```python
from build123d import *

# Parameters (mm, degrees)
BOSS_EXTRUDE1_DEPTH = 3.175
FILLET1_R           = 3.175
FILLET2_R           = 1.5875
SKETCH3_W           = 3.175
SKETCH3_H           = 12.7
SKETCH3_W_2         = 12.7
SKETCH3_H_2         = 3.175
SKETCH3_W_3         = 6.35
BOSS_EXTRUDE2_DEPTH = 3.175
CUT_EXTRUDE1_DEPTH  = 282.187550651
FILLET3_R           = 0.3175


with BuildPart() as part:
    # Sketch1 → Boss-Extrude1 (new body)
    with BuildSketch(Plane.XY):
        Polygon((-276.225, 0), (276.225, 0), (276.225, 31.496), (263.525, 31.496), (251.079, 19.05), (-251.079, 19.05), (-263.525, 31.496), (-276.225, 31.496), align=None)
    extrude(amount=BOSS_EXTRUDE1_DEPTH)

    # Fillet1
    fillet1_edges = [part.edges().sort_by_distance(p)[0] for p in [
        (-263.525, 31.496, 1.5875),
        (-251.079, 19.05, 1.5875),
        (251.079, 19.05, 1.5875),
        (263.525, 31.496, 1.5875),
    ]]
    fillet(fillet1_edges, radius=FILLET1_R)

    # Fillet2
    fillet2_edges = [part.edges().sort_by_distance(p)[0] for p in [
        (-276.225, 31.496, 1.5875),
        (276.225, 31.496, 1.5875),
        (276.225, 0, 1.5875),
        (-276.225, 0, 1.5875),
    ]]
    fillet(fillet2_edges, radius=FILLET2_R)

    # Sketch3 → Boss-Extrude2 (add)
    with BuildSketch(Plane.XY.offset(3.175)):
        with Locations((277.8125, 15.748)):
            Rectangle(SKETCH3_W, SKETCH3_H)
        with Locations((138.1125, -1.5875)):
            Rectangle(SKETCH3_W_2, SKETCH3_H_2)
        with Locations((3.175, -1.5875)):
            Rectangle(SKETCH3_W_3, SKETCH3_H_2)
    boss_extrude2 = extrude(amount=-BOSS_EXTRUDE2_DEPTH)

    # Mirror1: Boss-Extrude2 across plane
    add(boss_extrude2.mirror(Plane(origin=(0, 0, 0), x_dir=(0, 0, 1), z_dir=(1, 0, 0))))

    # Sketch4 → Cut-Extrude1 (cut, through all)
    with BuildSketch(Plane.XY.offset(3.175)):
        with BuildLine():
            Line((-276.225, 22.733), (-275.59, 22.733))
            ThreePointArc((-275.59, 22.733), (-275.2725, 22.4155), (-275.59, 22.098))
            Line((-275.59, 22.098), (-276.225, 22.098))
            ThreePointArc((-276.225, 22.098), (-276.5425, 22.4155), (-276.225, 22.733))
        make_face()
        with BuildLine():
            Line((-276.225, 9.398), (-275.59, 9.398))
            ThreePointArc((-275.59, 9.398), (-275.2725, 9.0805), (-275.59, 8.763))
            Line((-275.59, 8.763), (-276.225, 8.763))
            ThreePointArc((-276.225, 8.763), (-276.5425, 9.0805), (-276.225, 9.398))
        make_face()
        with BuildLine():
            Line((-145.0975, 0), (-145.0975, 0.635))
            ThreePointArc((-145.0975, 0.635), (-144.78, 0.9525), (-144.4625, 0.635))
            Line((-144.4625, 0.635), (-144.4625, 0))
            ThreePointArc((-144.4625, 0), (-144.78, -0.3175), (-145.0975, 0))
        make_face()
        with BuildLine():
            Line((-131.1275, 0.635), (-131.1275, 0))
            ThreePointArc((-131.1275, 0), (-131.445, -0.3175), (-131.7625, 0))
            Line((-131.7625, 0), (-131.7625, 0.635))
            ThreePointArc((-131.7625, 0.635), (-131.445, 0.9525), (-131.1275, 0.635))
        make_face()
        with BuildLine():
            Line((-6.985, 0), (-6.985, 0.635))
            ThreePointArc((-6.985, 0.635), (-6.6675, 0.9525), (-6.35, 0.635))
            Line((-6.35, 0.635), (-6.35, 0))
            ThreePointArc((-6.35, 0), (-6.6675, -0.3175), (-6.985, 0))
        make_face()
    cut_extrude1 = extrude(amount=-CUT_EXTRUDE1_DEPTH, mode=Mode.SUBTRACT)

    # Mirror2: Cut-Extrude1 across plane
    add(cut_extrude1.mirror(Plane(origin=(0, 0, 0), x_dir=(0, 0, 1), z_dir=(1, 0, 0))), mode=Mode.SUBTRACT)

    # Fillet3
    fillet3_edges = [part.edges().sort_by_distance(p)[0] for p in [
        (-279.4, 22.098, 1.5875),
        (-279.4, 9.398, 1.5875),
        (-144.4625, -3.175, 1.5875),
        (-131.7625, -3.175, 1.5875),
        (-6.35, -3.175, 1.5875),
        (-276.225, 22.733, 1.5875),
        (-276.225, 8.763, 1.5875),
        (-145.0975, 0, 1.5875),
        (-131.1275, 0, 1.5875),
        (-6.985, 0, 1.5875),
        (276.225, 22.733, 1.5875),
        (276.225, 8.763, 1.5875),
        (145.0975, 0, 1.5875),
        (131.1275, 0, 1.5875),
        (6.985, 0, 1.5875),
        (279.4, 22.098, 1.5875),
        (279.4, 9.398, 1.5875),
        (131.7625, -3.175, 1.5875),
        (144.4625, -3.175, 1.5875),
        (6.35, -3.175, 1.5875),
    ]]
    fillet(fillet3_edges, radius=FILLET3_R)


solid = part.part
```
Here's how the part is built. I have some questions about the finished solid (model axes, mm). A direction names the side the tool comes from. Coordinates: 2 decimals unless noted, no trailing zeros. Order: outer loops, then holes, each group sorted by start corner. A loop starts at its lowest first (then second) coordinate and runs counter-clockwise, first axis right, second up.
1) Imagine slicing it at A-A on x = -222.5. List the corners of the cut face in (y, z) for me (3 decimals), and give its area (3 significant figures).
2) I need wall thicknesses on line 1 (Y direction, x = -46, z = 1.05); line 2 (Y direction, x = 137.5, z = 1.2) (3 decimals); line 3 (X direction, y = 24, z = 2.65) (3 decimals). Which ranges of each line are inside material? Lowest first, please.
3) Will these pins go through, and if not, where does the flat tip stop? pin 1 (1.6 mm diameter, centred on x = -94.5, z = 2, fed in from -Y); pin 2 (1 mm diameter, centred on x = -208.5, z = 1, fed in from +Y); pin 3 (1.6 mm diameter, centred on x = -278, z = 2, fed in from -Y).
4) We'd pull the mould along X, two halves only. Please class faces 1 (the face through (-257.23, 25.2, 1.57)), 2 (the face through (4, 11, 0)): +X half, -X half, draft (parallel to the pull), parting line (faces both ways), or undercut.
5) Which directions (+Z, -Z, +X, -X, +Y, -Y) give clear straight access to the entire face, cutting with the end or side of a thin tool? Please do faces 3 (the face through (4, 11, 3.175)), 4 (the face through (257.38, 25.35, 1.57)).
Response values:
1. outline: (0, 0) - (19.05, 0) - (19.05, 3.175) - (0, 3.175) - close
1. area: 60.5 mm2
2. line 1: y = 0 to 19.05
2. line 2: y = -3.175 to 19.05
2. line 3: x = -276.225 to -256.029, 256.029 to 276.225
3. pin 1: stops at y = 0
3. pin 2: stops at y = 19.05
3. pin 3: stops at y = 9.4
4. face 1: undercut
4. face 2: draft
5. face 3: +Z, +X, -X, +Y, -Y
5. face 4: +Z, -Z, +Y
